Work out the finished part from the listing and answer in its coordinate system (mm). Face numbers are marked on the shaded views. A direction names the side the tool comes from. Give positions to 0.01 mm unless a question says otherwise; leave off trailing zeros. Order: outer loops, then holes, each group sorted by start corner. A loop starts at its lowest first (then second) coordinate and runs counter-clockwise, first axis right, second up. Notation, with made-up numbers: (35, 70) - (86, 70) arc R19 cw to (86, 92) - close; hole circle Ø9 at (63, 49.5). An arc over 180 degrees is marked (long way). Write each question's results on one line, items separated by ' | '.
from build123d import *

# Parameters (mm, degrees)
SKETCH1_R           = 2
BOSS_EXTRUDE2_DEPTH = 4
SKETCH1_2_R         = 2
BOSS_EXTRUDE3_DEPTH = 10


with BuildPart() as part:
    # Sketch1 → Boss-Extrude2 (new body)
    with BuildSketch(Plane.XY):
        with BuildLine():
            Line((-24, 3), (24, 3))
            ThreePointArc((24, 3), (27, 0), (24, -3))
            Line((24, -3), (-24, -3))
            ThreePointArc((-24, -3), (-27, 0), (-24, 3))
        make_face()
        with Locations((-24, 0)):
            Circle(SKETCH1_R, mode=Mode.SUBTRACT)
        with Locations((24, 0)):
            Circle(SKETCH1_R, mode=Mode.SUBTRACT)
        Circle(SKETCH1_R, mode=Mode.SUBTRACT)
    extrude(amount=BOSS_EXTRUDE2_DEPTH)

    # Sketch1<2> → Boss-Extrude3 (add)
    with BuildSketch(Plane.XY):
        Circle(SKETCH1_2_R)
    extrude(amount=BOSS_EXTRUDE3_DEPTH)


solid = part.part
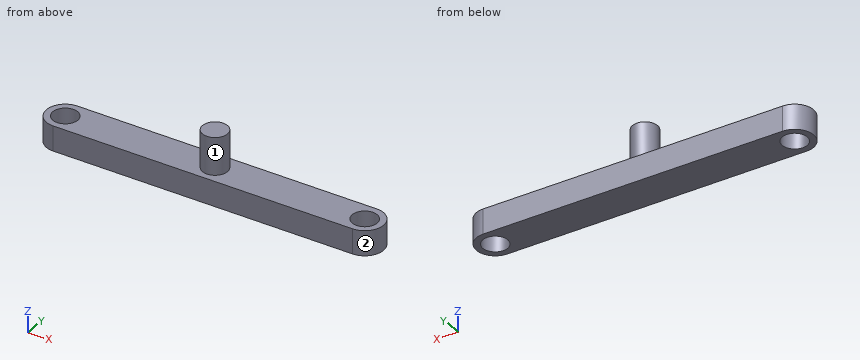
1. A tool of negligible diameter and unlimited length cuts with its end or side. For the marked faces 1 and 2, from which of +Z, -Z, +X, -X, +Y, -Y can it reach the whole face along a straight path? Write none if from no direction.
Answer list:
face 1: +Z | face 2: +Z, -Z, +X
2. A cutting plane is placed at D-D, the plane z = 6.5. Write down the section's boundary in (x, y).
Answer list:
outline: circle Ø4 at (0, 0)
3. A cutting plane is placed at B-B, the plane x = 0. Write down the section's boundary in (y, z).
Answer list:
outline: (-3, 0) - (3, 0) - (3, 4) - (2, 4) - (2, 10) - (-2, 10) - (-2, 4) - (-3, 4) - close
4. A cutting plane is placed at A-A, the plane y = 0. Write down the section's boundary in (x, z), then the cut area to 3 significant figures.
Answer list:
outline: (-27, 0) - (-26, 0) - (-26, 4) - (-27, 4) - close; (-22, 0) - (22, 0) - (22, 4) - (2, 4) - (2, 10) - (-2, 10) - (-2, 4) - (-22, 4) - close; (26, 0) - (27, 0) - (27, 4) - (26, 4) - close | area: 208 mm^2
5. Straight lines are drawn through the part: line 1 (Y direction, x = 24, z = 1.1); line 2 (X direction, y = -1.3, z = 1); line 3 (X direction, y = 1.45, z = 0.75). For each, find the intervals that lie inside material, in ascending order. Write a range as [from, to].
Answer list:
line 1: [-3, -2], [2, 3] | line 2: [-26.7, -25.52], [-22.48, 22.48], [25.52, 26.7] | line 3: [-26.63, -25.38], [-22.62, 22.62], [25.38, 26.63]
6. Given P1, Ø1, axis at x = -10.5, y = -2.5, coming from the +Z side, flat-ended and moving along its own axis, determine where the tip first touches the part or whether it passes through.
Answer list:
P1: z = 4
7. A cutting plane is placed at C-C, the plane z = 2. Write down the section's boundary in (x, y).
Answer list:
outline: (-24, -3) - (24, -3) arc R3 ccw to (24, 3) - (-24, 3) arc R3 ccw to start; hole circle Ø4 at (-24, 0); hole circle Ø4 at (24, 0)
